from build123d import *

# Parameters (mm, degrees)
SKETCH1_R           = 1
SKETCH1_R_2         = 2.75
BOSS_EXTRUDE1_DEPTH = 2
SKETCH2_W           = 15
SKETCH2_H           = 4
BOSS_EXTRUDE2_DEPTH = 20
SKETCH3_R           = 2
CUT_EXTRUDE1_DEPTH  = 20


with BuildPart() as part:
    # Sketch1 → Boss-Extrude1 (new body)
    with BuildSketch(Plane(origin=(0, 0, 0), x_dir=(1, 0, 0), z_dir=(0, 1, 0))):
        with BuildLine():
            Line((0, -26), (0, 0))
            Line((0, 0), (-32.806184042, 0))
            Line((-32.806184042, 0), (-47.806184042, 0))
            Line((-47.806184042, 0), (-108.64, 0))
            Line((-108.64, 0), (-108.64, -26))
            Line((-108.64, -26), (-84.372050808, -26))
            ThreePointArc((-84.372050808, -26), (-83.15763809, -23.068148347), (-80.64, -25))
            ThreePointArc((-80.64, -25), (-80.708148347, -25.51763809), (-80.907949192, -26))
            Line((-80.907949192, -26), (-27.732050808, -26))
            ThreePointArc((-27.732050808, -26), (-26.51763809, -23.068148347), (-24, -25))
            ThreePointArc((-24, -25), (-24.068148347, -25.51763809), (-24.267949192, -26))
            Line((-24.267949192, -26), (0, -26))
        make_face()
        with Locations((-77.82, -21)):
            Circle(SKETCH1_R, mode=Mode.SUBTRACT)
        with Locations((-98.64, -13)):
            Circle(SKETCH1_R_2, mode=Mode.SUBTRACT)
        with Locations((-77.82, -5)):
            Circle(SKETCH1_R, mode=Mode.SUBTRACT)
        with Locations((-30.82, -13)):
            Circle(SKETCH1_R, mode=Mode.SUBTRACT)
        with Locations((-10, -13)):
            Circle(SKETCH1_R_2, mode=Mode.SUBTRACT)
    extrude(amount=BOSS_EXTRUDE1_DEPTH)

    # Sketch2 → Boss-Extrude2 (add)
    with BuildSketch(Plane(origin=(0, 2, 0), x_dir=(1, 0, 0), z_dir=(0, 1, 0))):
        with Locations((-39.138364189, -2)):
            Rectangle(SKETCH2_W, SKETCH2_H)
    extrude(amount=BOSS_EXTRUDE2_DEPTH)

    # Sketch3 → Cut-Extrude1 (cut)
    with BuildSketch(Plane.XY.offset(4)):
        with Locations((-39.138364189, 18.622728592)):
            Circle(SKETCH3_R)
    extrude(amount=-CUT_EXTRUDE1_DEPTH, mode=Mode.SUBTRACT)


solid = part.part
The listing builds one solid part. Answer for the finished solid, in the listing's coordinates (mm). A direction names the side the tool comes from. Round coordinates to 2 decimals unless told otherwise and drop trailing zeros. Loops run counter-clockwise (first coordinate to the right, second up) from the corner with the lowest first, then second, coordinate; pieces in that order, holes last. Notation, with made-up numbers: M 13.25,56.25 L 20.25,56.25 A10 cw 20.25,62.25 Z; hole C -27,40.5 d9. An arc over 180 degrees is marked long. Return JSON: item names as keys, results as strings.
Q1. Find section B-B, the plane z = 5. Determine the outline of the cut face in (x, y), plus the area to 3 significant figures.
Results list:
{"outline": "M -108.64,0 L -78.82,0 L -78.82,2 L -108.64,2 Z; M -76.82,0 L 0,0 L 0,2 L -76.82,2 Z", "area": "213 mm2"}
Q2. Find section D-D, the plane y = 8.25. Determine the outline of the cut face in (x, z), plus the area to 3 significant figures.
Results list:
{"outline": "M -46.64,0 L -31.64,0 L -31.64,4 L -46.64,4 Z", "area": "60.0 mm2"}
Q3. Which of the six approach directions +Z, -Z, +X, -X, +Y, -Y give full straight-line access (tool end or side, diameter ignored) to faces 4 (the face through (-39, 12, 4)), 5 (the face through (-46.638, 12, 2)), 6 (the face through (-31.638, 12, 2))?
Results list:
{"face 4": "+Z, +X, -X, +Y", "face 5": "+Z, -Z, -X, +Y", "face 6": "+Z, -Z, +X, +Y"}
Q4. Each of these flat-tipped pins is pushed along its axis until it touches: pin 1 Ø1.2 at (x, z) = (-77.82, 21) entering from +Y; pin 2 Ø7.5 at (x, y) = (-41, 8) entering from +Z; pin 3 Ø4.5 at (x, z) = (-82.64, 25) entering from +Y; pin 4 Ø3 at (y, z) = (8, 2) entering from +X. Where does it stop, or does it pass through?
Results list:
{"pin 1": "passes through", "pin 2": "stops at z = 4", "pin 3": "stops at y = 2", "pin 4": "stops at x = -31.64"}
Q5. Find section A-A, the plane x = -98.64. Determine the outline of the cut face in (y, z).
Results list:
{"outline": "M 0,0 L 2,0 L 2,10.25 L 0,10.25 Z; M 0,15.75 L 2,15.75 L 2,26 L 0,26 Z"}
Q6. The mould has two halves that part along Z. Classify faces 1 (the face through (-46, 7, 0)), 2 (the face through (-31.61, 0.99, 13.61)), 3 (the face through (-39, 22, 2)): released by +Z, released by -Z, zero draft, split by the parting line, or undercut.
Results list:
{"face 1": "released by -Z", "face 2": "undercut", "face 3": "zero draft"}
Q7. Find the intervals of material crossed by line 1 along X through (y, z) = (0.4, 13); line 2 along X through (y, z) = (1.65, 25); line 3 along Z through (x, y) = (-98.64, 1.3), in increasing order. Write a range as from..to.
Results list:
{"line 1": "x = -108.64..-101.39, -95.89..-31.82, -29.82..-12.75, -7.25..0", "line 2": "x = -108.64..-84.64, -80.64..-28, -24..0", "line 3": "z = 0..10.25, 15.75..26"}
Q8. Find section C-C, the plane z = 13. Determine the outline of the cut face in (x, y), plus the area to 3 significant figures.
Results list:
{"outline": "M -108.64,0 L -101.39,0 L -101.39,2 L -108.64,2 Z; M -95.89,0 L -31.82,0 L -31.82,2 L -95.89,2 Z; M -29.82,0 L -12.75,0 L -12.75,2 L -29.82,2 Z; M -7.25,0 L 0,0 L 0,2 L -7.25,2 Z", "area": "191 mm2"}
